Source: CAD feature listing. Evaluate the final solid. Frame: model axes, mm. Round coordinates to 2 decimals unless told otherwise and drop trailing zeros. Loops run counter-clockwise (first coordinate to the right, second up) from the corner with the lowest first, then second, coordinate; pieces in that order, holes last. Notation, with made-up numbers: (-7.75, -39.5) - (16.25, -39.5) arc R30 cw to (16.25, -1.5) - close; hole circle Ø10 at (-6.5, 44.5). An arc over 180 degrees is marked (long way). One line per question, with ' | ' between items. Start each with the question number.
1. Cut plane A-A (y = 28). Return loops of the section in (x, z).
2. Cut plane C-C (z = 0.5). State how many separate pieces and enclosed holes the cut face has, then the cut area to 3 significant figures.
3. Pin query (flat end, axial travel): pin 1 (6 mm diameter, centred on x = 21.5, y = -4.5, fed in from -Z); pin 2 (0.8 mm diameter, centred on y = 78.5, z = 0.5, fed in from -X). Return the tip coordinate at first contact, or that it passes through.
4. Cut plane D-D (x = 166). Return loops of the section in (y, z), then the cut area to 3 significant figures.
5. Cut plane B-B (x = 33). Return loops of the section in (y, z), then the cut area to 3 significant figures.
6. Ray query, line 1 (X direction, y = 33, z = 0.75); line 2 (X direction, y = 49, z = 0.75); line 3 (Y direction, x = 66.5, z = 1.45). Return the intervals inside material, ascending.
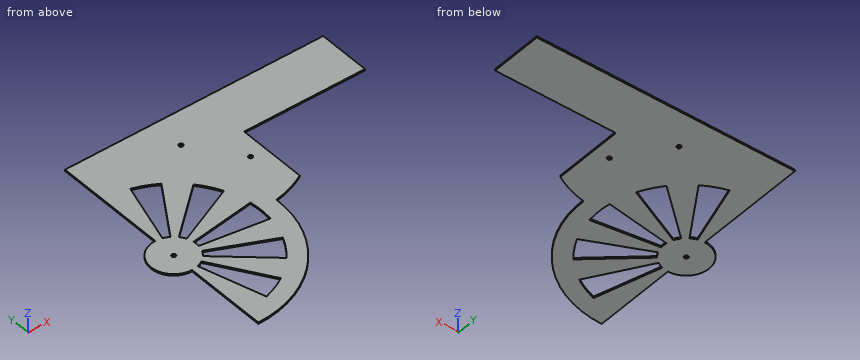
```python
from build123d import *

# Parameters (mm, degrees)
SKETCH1_R           = 2
BOSS_EXTRUDE1_DEPTH = 1.5
CUT_EXTRUDE1_DEPTH  = 2.5


with BuildPart() as part:
    # Sketch1 → Boss-Extrude1 (new body)
    with BuildSketch(Plane.XY):
        with BuildLine():
            Line((0, 130), (0, 22))
            ThreePointArc((0, 22), (-22, 0), (0, -22))
            Line((0, -22), (0, -101.426173946))
            ThreePointArc((0, -101.426173946), (72.567414345, -70.860702344), (101.397454872, 2.413484395))
            ThreePointArc((101.397454872, 2.413484395), (117.671962719, 6.534414164), (132.983960448, 13.418046445))
            Line((132.983960448, 13.418046445), (132.983960448, 80))
            Line((132.983960448, 80), (250, 80))
            Line((250, 80), (250, 130))
            Line((250, 130), (0, 130))
        make_face()
        Circle(SKETCH1_R, mode=Mode.SUBTRACT)
        with Locations((85.977020164, 97.508727834)):
            Circle(SKETCH1_R, mode=Mode.SUBTRACT)
        with Locations((118.232097827, 54.047858824)):
            Circle(SKETCH1_R, mode=Mode.SUBTRACT)
    extrude(amount=BOSS_EXTRUDE1_DEPTH)

    # Sketch2 → Cut-Extrude1 (cut, through all)
    with BuildSketch(Plane.XY.offset(1.5)):
        with BuildLine():
            Line((6.198116251, -21.10884542), (23.947267332, -81.556902757))
            ThreePointArc((23.947267332, -81.556902757), (35.310276105, -77.318719605), (45.954469484, -71.506550291))
            Line((45.954469484, -71.506550291), (11.894097984, -18.507577722))
            ThreePointArc((11.894097984, -18.507577722), (9.139130286, -20.011903898), (6.198116251, -21.10884542))
        make_face()
        with BuildLine():
            Line((16.626490636, -14.406936147), (64.23871382, -55.663162385))
            ThreePointArc((64.23871382, -55.663162385), (71.506550291, -45.954469484), (77.318719605, -35.310276105))
            Line((77.318719605, -35.310276105), (20.011903898, -9.139130286))
            ThreePointArc((20.011903898, -9.139130286), (18.507577722, -11.894097984), (16.626490636, -14.406936147))
        make_face()
        with BuildLine():
            Line((21.776071721, -3.130926442), (84.13482256, -12.096761253))
            ThreePointArc((84.13482256, -12.096761253), (85, 0), (84.13482256, 12.096761253))
            Line((84.13482256, 12.096761253), (21.776071721, 3.130926442))
            ThreePointArc((21.776071721, 3.130926442), (22, 0), (21.776071721, -3.130926442))
        make_face()
        with BuildLine():
            Line((20.011903898, 9.139130286), (77.318719605, 35.310276105))
            ThreePointArc((77.318719605, 35.310276105), (71.506550291, 45.954469484), (64.23871382, 55.663162385))
            Line((64.23871382, 55.663162385), (16.626490636, 14.406936147))
            ThreePointArc((16.626490636, 14.406936147), (18.507577722, 11.894097984), (20.011903898, 9.139130286))
        make_face()
        with BuildLine():
            Line((11.894097984, 18.507577722), (45.954469484, 71.506550291))
            ThreePointArc((45.954469484, 71.506550291), (35.310276105, 77.318719605), (23.947267332, 81.556902757))
            Line((23.947267332, 81.556902757), (6.198116251, 21.10884542))
            ThreePointArc((6.198116251, 21.10884542), (9.139130286, 20.011903898), (11.894097984, 18.507577722))
        make_face()
    extrude(amount=-CUT_EXTRUDE1_DEPTH, mode=Mode.SUBTRACT)


solid = part.part
```
Answers follow:
1) outline: (0, 0) - (8.22, 0) - (8.22, 1.5) - (0, 1.5) - close; (17.99, 0) - (32.31, 0) - (32.31, 1.5) - (17.99, 1.5) - close; (61.31, 0) - (132.98, 0) - (132.98, 1.5) - (61.31, 1.5) - close
2) separate pieces: 1 | enclosed holes: 8 | area: 26,900 mm2
3) pin 1: stops at z = 0 | pin 2: stops at x = 0
4) outline: (80, 0) - (130, 0) - (130, 1.5) - (80, 1.5) - close | area: 75.0 mm2
5) outline: (-95.91, 0) - (-78.33, 0) - (-78.33, 1.5) - (-95.91, 1.5) - close; (-51.35, 0) - (-28.59, 0) - (-28.59, 1.5) - (-51.35, 1.5) - close; (-15.07, 0) - (-4.74, 0) - (-4.74, 1.5) - (-15.07, 1.5) - close; (4.74, 0) - (15.07, 0) - (15.07, 1.5) - (4.74, 1.5) - close; (28.59, 0) - (51.35, 0) - (51.35, 1.5) - (28.59, 1.5) - close; (78.33, 0) - (130, 0) - (130, 1.5) - (78.33, 1.5) - close | area: 203 mm2
6) line 1: x = 0 to 9.69, 21.21 to 38.08, 72.26 to 132.98 | line 2: x = 0 to 14.39, 31.49 to 56.55, 69.46 to 132.98 | line 3: y = -76.58 to -52.94, -30.37 to -9.56, 9.56 to 30.37, 52.94 to 130
